CAD build for the part. Positions are in the model's coordinates, mm. Face numbers are marked on the shaded views. A direction names the side the tool comes from. Give positions to 0.01 mm unless a question says otherwise; leave off trailing zeros. Loops run counter-clockwise (first coordinate to the right, second up) from the corner with the lowest first, then second, coordinate; pieces in that order, holes last.
```python
from build123d import *

# Parameters (mm, degrees)
F0_R         = 8.85
F1_DEPTH     = 1.4
F2_R         = 7.175
F2_R_2       = 6.275
F3_DEPTH     = 4
F5_W         = 2.85
F5_H         = 4
F6_DEPTH     = 25
F7_R         = 4.4
F8_DEPTH     = 1.27
F10_W        = 1.7
F10_H        = 1.25
F11_DEPTH    = 0.6
F12_W        = 12.45
F12_H        = 1.85
F13_DEPTH    = 0.8
F14_T1_DEPTH = 6.7489794856
F15_R        = 0.25


# Not quite as in the source:
# - a fillet or chamfer that OpenCascade refuses, or shapes differently, is made with other operations: its cross-section is extruded or revolved along the edge and cut away or added
# - a pattern or mirror of a feature is missing from the dataset's text; its kind, count and spacing are read off the source's solid


with BuildPart() as f1:
    # F0 (on Top) → F1 (new body)
    with BuildSketch(Plane.XY):
        Circle(F0_R)
    extrude(amount=F1_DEPTH)

    # F2 (on face) → F3 (join)
    with BuildSketch(Plane.XY.offset(1.4)):
        Circle(F2_R)
        Circle(F2_R_2, mode=Mode.SUBTRACT)
    extrude(amount=F3_DEPTH)

    # F5 (on offset) → F6 (cut)
    with BuildSketch(Plane.YZ.offset(7.175)):
        with Locations((0, 3.4)):
            Rectangle(F5_W, F5_H)
    extrude(amount=-F6_DEPTH, mode=Mode.SUBTRACT)

    # F7 (on face) → F8 (join)
    with BuildSketch(Plane.XY.offset(1.4)):
        Circle(F7_R)
    extrude(amount=F8_DEPTH)

    # F10 (on offset) → F11 (join, symmetric)
    with BuildSketch(Plane.XZ.offset(7.175)):
        with Locations((0, 4.275)):
            Rectangle(F10_W, F10_H)
    f11 = extrude(amount=F11_DEPTH, both=True)

    # F11_copies: F11 across plane
    add(f11.mirror(Plane.ZX))

    # F12 (on face) → F13 (cut)
    with BuildSketch(Plane(origin=(0, 0, 0), x_dir=(1, 0, 0), z_dir=(0, 0, -1))):
        Rectangle(F12_W, F12_H)
    extrude(amount=-F13_DEPTH, mode=Mode.SUBTRACT)

    # F14: fillet of radius 1 on 2 edges, made by hand

    # F14_s2 → F14_t1 (join)
    with BuildSketch(Plane.XZ.offset(-3.3744897428)):
        with BuildLine():
            ThreePointArc((-6.225, 0), (-5.8776596349, 0.5745966692), (-5.2452041029, 0.8))
            Line((-5.2452041029, 0.8), (-6.225, 0.8))
            Line((-6.225, 0.8), (-6.225, 0))
        make_face()
        with BuildLine():
            ThreePointArc((6.225, 0), (5.8776596349, 0.5745966692), (5.2452041029, 0.8))
            Line((5.2452041029, 0.8), (6.225, 0.8))
            Line((6.225, 0.8), (6.225, 0))
        make_face()
    extrude(amount=F14_T1_DEPTH)

    # F15
    f15_edges = [f1.edges().sort_by_distance(p)[0] for p in [
        (0, 6.275, 1.4),
        (6.571562, 1.425, 1.4),
        (-6.571562, 1.425, 1.4),
        (0, 7.175, 1.4),
        (-4.4, 0, 1.4),
        (-6.571562, -1.425, 1.4),
        (6.571562, -1.425, 1.4),
        (0, -7.175, 1.4),
        (0, -6.275, 1.4),
    ]]
    fillet(f15_edges, radius=F15_R)


solid = f1.part
```
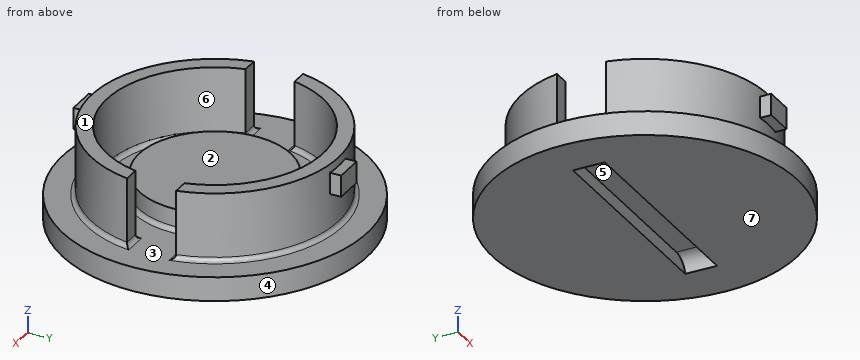
1. Tool access for the marked faces 5, 6 and 7: list every direction of +Z, -Z, +X, -X, +Y, -Y with a clear straight run to the whole face (end or side of a thin tool).
Responses:
face 5: -Z
face 6: +Z
face 7: -Z, +X, -X, +Y, -Y
2. Saw through at C-C, the plane z = 1.15. List the corners of the cut face in (x, y).
Responses:
outline: circle Ø17.7 at (0, 0)
3. Saw through at A-A, the plane y = 0. List the corners of the cut face in (x, z) (3 decimals), and give its area (3 significant figures).
Responses:
outline: (-8.85, 0) - (-6.225, 0) arc R1 cw to (-5.245, 0.8) - (5.245, 0.8) arc R1 cw to (6.225, 0) - (8.85, 0) - (8.85, 1.4) - (4.65, 1.4) arc R0.25 cw to (4.4, 1.65) - (4.4, 2.67) - (-4.4, 2.67) - (-4.4, 1.65) arc R0.25 cw to (-4.65, 1.4) - (-8.85, 1.4) - close
area: 26.4 mm2
4. Drop flat-ended pins along their axis: pin 1 (3 mm diameter, centred on x = 0.5, z = 4, fed in from +Y) (3 decimals); pin 2 (8 mm diameter, centred on x = 0, y = -2, fed in from +Z); pin 3 (0.7 mm diameter, centred on x = -6.5, z = 3, fed in from +Y). Give the stop position or say it passes through.
Responses:
pin 1: stops at y = 7.775
pin 2: stops at z = 2.67
pin 3: stops at y = 3.7
5. Probe line 1 along X through (y, z) = (-4, 2.05); line 2 along Y through (x, z) = (2, 1.9); line 3 along Y through (x, z) = (-3, 1.65). List the from-to ranges inside material, lowest first.
Responses:
line 1: x = -5.96 to -4.83, -1.83 to 1.83, 4.83 to 5.96
line 2: y = -6.89 to -5.95, -3.92 to 3.92, 5.95 to 6.89
line 3: y = -6.52 to -5.51, -3.22 to 3.22, 5.51 to 6.52
6. Pull direction Y, two halves, no side cores. Call the marked faces 1, 2, 3 and 4: released by +Y, released by -Y, zero draft, split by the parting line, or undercut.
Responses:
face 1: zero draft
face 2: undercut
face 3: undercut
face 4: split by the parting line
